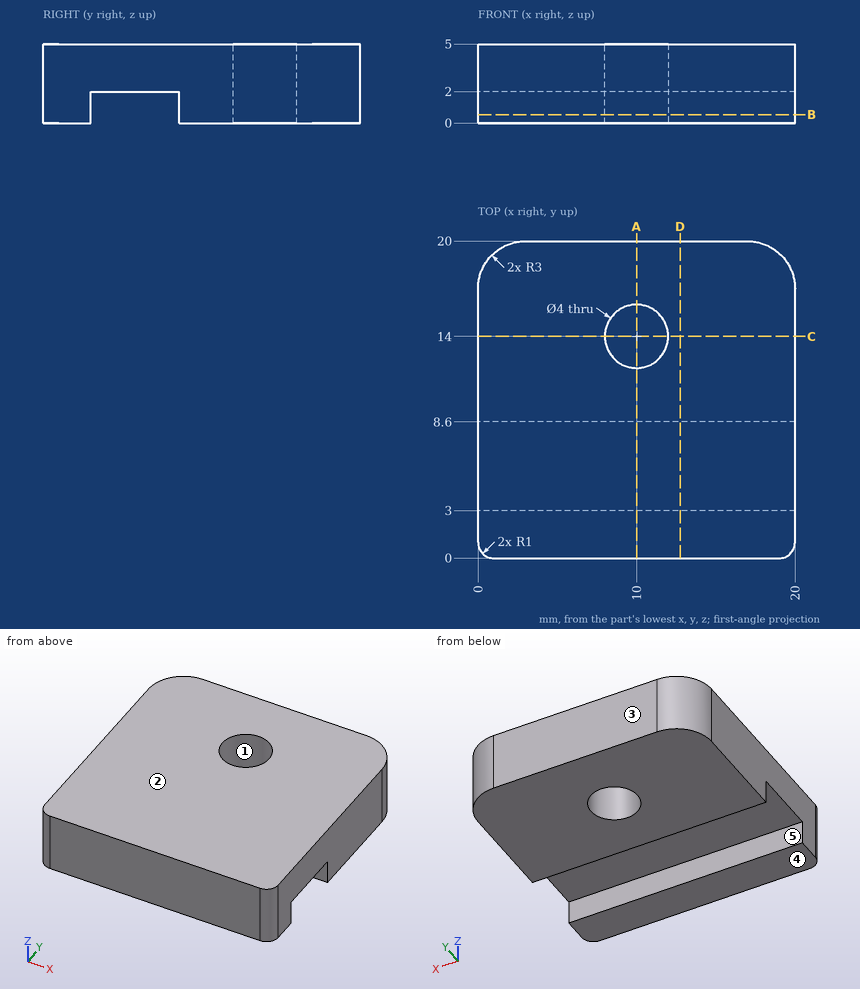
Check sheet for the drawn part. Datum: minimum x, y, z corner. Units: mm. A direction names the side the tool comes from. Round coordinates to 2 decimals unless told otherwise and drop trailing zeros. Loops run counter-clockwise (first coordinate to the right, second up) from the corner with the lowest first, then second, coordinate; pieces in that order, holes last. Notation, with made-up numbers: (-13, -28.75) - (40, -28.75) arc R10 cw to (40, -9.75) - close; hole circle Ø2 at (35.5, 21.5). An arc over 180 degrees is marked (long way). Use one line per item in the form item = value.
1. Section check A-A on x = 10. Record the cut outline in (y, z), and give its area (3 significant figures).
A:
outline = (0, 0) - (3, 0) - (3, 2) - (8.6, 2) - (8.6, 0) - (12, 0) - (12, 5) - (0, 5) - close; (16, 0) - (20, 0) - (20, 5) - (16, 5) - close
area = 68.8 mm²
2. Section check B-B on z = 0.55. Record the cut outline in (x, y).
A:
outline = (0, 1) arc R1 ccw to (1, 0) - (19, 0) arc R1 ccw to (20, 1) - (20, 3) - (0, 3) - close; (0, 8.6) - (20, 8.6) - (20, 17) arc R3 ccw to (17, 20) - (3, 20) arc R3 ccw to (0, 17) - close; hole circle Ø4 at (10, 14)
3. Gauge pin test, flat end, axial feed: pin 1 Ø3 at (x, y) = (11, 5.5) entering from -Z. Record the tip position at first contact, or that the pin passes through.
A:
pin_1 = 2
4. Section check D-D on x = 12.75. Record the cut outline in (y, z), and give its area (3 significant figures).
A:
outline = (0, 0) - (3, 0) - (3, 2) - (8.6, 2) - (8.6, 0) - (20, 0) - (20, 5) - (0, 5) - close
area = 88.8 mm²
5. Draft check along Y on the marked faces 1, 2 and 3. Enter one of: pulls with the +Y half, pulls with the -Y half, needs draft (parallel to the pull), parting line crosses it, or undercut.
A:
face_1 = undercut
face_2 = needs draft
face_3 = pulls with the +Y half
6. Scan lines: probe 1 along Y at (x, z) = (10, 1.9); probe 2 along Y at (x, z) = (10, 3.8); probe 3 along Y at (x, z) = (14.5, 1.5). Record each from-to range of solid material in increasing order.
A:
probe_1 = 0 to 3, 8.6 to 12, 16 to 20
probe_2 = 0 to 12, 16 to 20
probe_3 = 0 to 3, 8.6 to 20
7. Access from +Z, -Z, +X, -X, +Y, -Y to the whole of each face (thin tool, end or side, straight path). Record for the marked faces 4 and 5.
A:
face_4 = -Z, +X, -X, +Y, -Y
face_5 = -Z, +X, -X
8. Section check C-C on y = 14. Record the cut outline in (x, z), and give its area (3 significant figures).
A:
outline = (0, 0) - (8, 0) - (8, 5) - (0, 5) - close; (12, 0) - (20, 0) - (20, 5) - (12, 5) - close
area = 80.0 mm²
